Design review of the part built by this model. Coordinates are the model's own, in mm. Face numbers are marked on the shaded views. A direction names the side the tool comes from. Give positions to 0.01 mm unless a question says otherwise; leave off trailing zeros. Loops run counter-clockwise (first coordinate to the right, second up) from the corner with the lowest first, then second, coordinate; pieces in that order, holes last. Notation, with made-up numbers: (-27.5, -13.5) -> (12.5, -13.5) arc R13 cw to (12.5, 2.5) -> close; hole circle Ø8 at (27, 7.25). An arc over 180 degrees is marked (long way). Use a Markdown table: item, result. Add a question column.
1. For pin 1 Ø4.5 at (y, z) = (2.5, 4) entering from +X; pin 2 Ø1 at (x, z) = (1.5, 3.5) entering from +Y; pin 3 Ø3 at (x, z) = (1, 6) entering from +Y, all flat-tipped, find the tip position at first contact; note any pin that passes through.
2. Add section A-A (z = 0.5). State the section outline as (x, y) points.
3. Add section C-C (x = -6.75). State the section outline as (y, z) points.
4. Add section B-B (y = 12.5). State the section outline as (x, z) points.
5. For the marked faces 1, 2, 3, 4 and 5, list the 3-axis set-ups (+Z, -Z, +X, -X, +Y, -Y) from which the entire face can be reached by the end or side of a thin tool; tool diameter is ignored.
6. Draft analysis for pull direction X (two halves, no side actions). For the marked faces 6, 7 and 8, state which applies: pulls with the +X half, pulls with the -X half, needs draft (parallel to the pull), parting line crosses it, or undercut.
7. To check wall thickness, follow line 1 (Y direction, x = 0, z = 5.5); line 2 (X direction, y = 8, z = 2.25); line 3 (Y direction, x = 1, z = 0.5). State the ranges of each line that lie inside material, in increasing order.
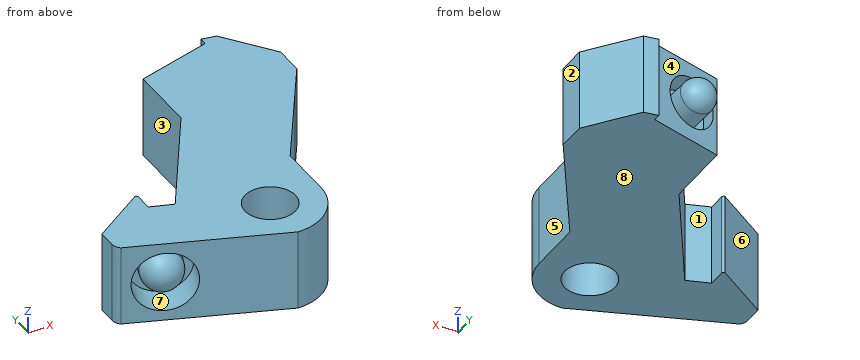
```python
from build123d import *

# Parameters (mm, degrees)
SKETCH_1_R          = 2.5
EXTRUDE_1_DEPTH     = 8
SKETCH_5_R          = 3
CUT_EXTRUDE_2_DEPTH = 3
SKETCH_7_R          = 2
EXTRUDE_3_DEPTH     = 3
FILLET_5_R          = 2
SKETCH_9_R          = 2.55
CUT_EXTRUDE_3_DEPTH = 1.5
SKETCH_10_R         = 1.7
EXTRUDE_4_DEPTH     = 5
FILLET_6_R          = 1.7


with BuildPart() as part:
    # 스케치1 → 보스-돌출1 (new body)
    with BuildSketch(Plane.XY):
        with BuildLine():
            Line((6.875581969, 24), (-0.451148657, 21.875531488))
            Line((-0.451148657, 21.875531488), (-0.451148657, 15.101495802))
            Line((-0.451148657, 15.101495802), (-7.258120431, 3.851310171))
            Line((-7.258120431, 3.851310171), (-9.5, 4.598603361))
            Line((-9.5, 4.598603361), (-9.5, 6.358960817))
            ThreePointArc((-9.5, 6.358960817), (-9.571850512, 6.512511163), (-9.735777088, 6.555734799))
            Line((-9.735777088, 6.555734799), (-15, 2.937976957))
            Line((-15, 2.937976957), (-15, 1.111926907))
            ThreePointArc((-15, 1.111926907), (-14.889635684, 0.655255963), (-14.582903299, 0.299385373))
            Line((-14.582903299, 0.299385373), (0, -5))
            ThreePointArc((0, -5), (3.535533906, -3.535533906), (5, 0))
            Line((5, 0), (5, 3.83484861))
            Line((5, 3.83484861), (5, 5.464934457))
            Line((5, 5.464934457), (10.112329073, 13.81338505))
            Line((10.112329073, 13.81338505), (11.945796901, 16.807444187))
            Line((11.945796901, 16.807444187), (11.945796901, 19.676308628))
            Line((11.945796901, 19.676308628), (8.295575886, 24.508809453))
            Line((8.295575886, 24.508809453), (6.875581969, 24.728164545))
            Line((6.875581969, 24.728164545), (6.875581969, 24))
        make_face()
        Circle(SKETCH_1_R, mode=Mode.SUBTRACT)
    extrude(amount=EXTRUDE_1_DEPTH)

    # 스케치5 → 컷-돌출2 (cut)
    with BuildSketch(Plane(origin=(-1.605029546, -4.416736851, 0), x_dir=(0.9398656128397294, -0.34154447704713375, 0), z_dir=(-0.34154447704713375, -0.9398656128397295, 0))):
        with Locations((-9.929236479, 4)):
            Circle(SKETCH_5_R)
    extrude(amount=-CUT_EXTRUDE_2_DEPTH, mode=Mode.SUBTRACT)

    # 스케치7 → 보스-돌출3 (add)
    with BuildSketch(Plane(origin=(-0.580396115, -1.597140012, 0), x_dir=(0.9398656128397294, -0.34154447704713387, 0), z_dir=(-0.34154447704713387, -0.9398656128397294, 0))):
        with Locations((-9.929236479, 4)):
            Circle(SKETCH_7_R)
    extrude(amount=EXTRUDE_3_DEPTH)

    # 필렛5
    fillet_5_edges = [part.edges().sort_by_distance(p)[0] for p in [
        (-12.8169087, -0.342372016, 4),
    ]]
    fillet(fillet_5_edges, radius=FILLET_5_R)

    # 스케치9 → 컷-돌출3 (cut, symmetric)
    with BuildSketch(Plane(origin=(-0.449080246, 21.87557395, 0), x_dir=(-0.9997893498603082, -0.02052451962658901, 0), z_dir=(0.02052451962658901, -0.9997893498603082, 0))):
        with Locations(Location((-2.997931152, -4, 0), (0, 0, 180))):
            Circle(SKETCH_9_R)
    extrude(amount=CUT_EXTRUDE_3_DEPTH, both=True, mode=Mode.SUBTRACT)

    # 스케치10 → 보스-돌출4 (add)
    with BuildSketch(Plane(origin=(-0.418293466, 20.375889925, 0), x_dir=(0.9997893498603082, 0.020524519626589015, 0), z_dir=(-0.020524519626589015, 0.9997893498603082, 0))):
        with Locations((2.997931152, -4)):
            Circle(SKETCH_10_R)
    extrude(amount=EXTRUDE_4_DEPTH)

    # 필렛6
    fillet_6_edges = [part.edges().sort_by_distance(p)[0] for p in [
        (0.776741679, 25.401476088, 4),
    ]]
    fillet(fillet_6_edges, radius=FILLET_6_R)


solid = part.part
```
Taken from the geometry:
| question | item | result |
|---|---|---|
| 1 | pin 1 | stops at x = 5 |
| 1 | pin 2 | stops at y = 25.32 |
| 1 | pin 3 | stops at y = 25.11 |
| 2 | outline | (-15, 1.11) arc R1 ccw to (-14.58, 0.3) -> (0, -5) arc R5 ccw to (5, 0) -> (5, 5.46) -> (11.95, 16.81) -> (11.95, 19.68) -> (8.3, 24.51) -> (6.88, 24.73) -> (6.88, 24) -> (-0.45, 21.88) -> (-0.45, 15.1) -> (-7.26, 3.85) -> (-9.5, 4.6) -> (-9.5, 6.36) arc R0.2 ccw to (-9.74, 6.56) -> (-15, 2.94) -> close; hole circle Ø5 at (0, 0) |
| 3 | outline | (-2.55, 0) -> (4.69, 0) -> (4.69, 8) -> (-2.55, 8) -> close |
| 4 | outline | (-2.03, 0) -> (9.31, 0) -> (9.31, 8) -> (-2.03, 8) -> close |
| 5 | face 1 | +Z, -Z, +Y |
| 5 | face 2 | +Z, -Z, +X, +Y, -Y |
| 5 | face 3 | +Z, -Z, -X, +Y |
| 5 | face 4 | +Y |
| 5 | face 5 | +Z, -Z, +X, -Y |
| 6 | face 6 | pulls with the -X half |
| 6 | face 7 | undercut |
| 6 | face 8 | needs draft |
| 7 | line 1 | y = -5 to -2.5, 2.5 to 22.01 |
| 7 | line 2 | x = -4.75 to 6.55 |
| 7 | line 3 | y = -4.9 to -2.29, 2.29 to 22.3 |
